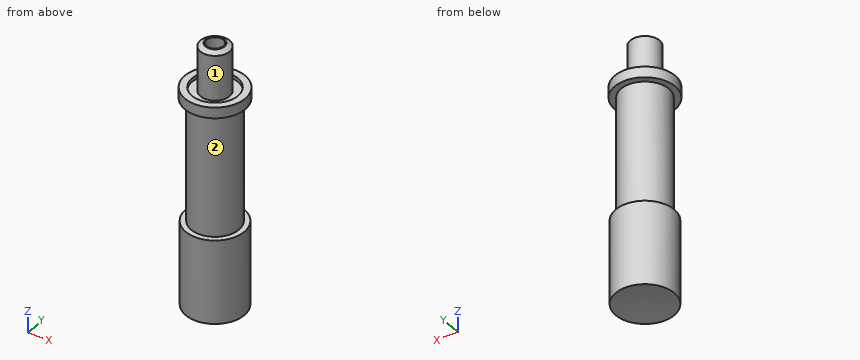
from build123d import *

# Parameters (mm, degrees)
CUT_EXTRUDE1_START = -10
SKETCH2_R          = 5
SKETCH2_R_2        = 2.45
CUT_EXTRUDE1_DEPTH = 10


with BuildPart() as part:
    # Sketch1 → Revolve1 (revolve)
    with BuildSketch(Plane(origin=(0, 0, 0), x_dir=(1, 0, 0), z_dir=(0, 1, 0))):
        with BuildLine():
            Line((0, 24.784048752), (0, 10.1))
            Line((0, 10.1), (0.6, 10.1))
            Line((0.6, 10.1), (0.7, 3.1))
            Line((0.7, 3.1), (0.79197487, 3.1))
            Line((0.79197487, 3.1), (1.225, 3.350011099))
            Line((1.225, 3.350011099), (1.225, 7.1))
            Line((1.225, 7.1), (1.925, 7.1))
            Line((1.925, 7.1), (1.925, 6.8))
            Line((1.925, 6.8), (2.525, 6.8))
            Line((2.525, 6.8), (2.525, 7.7))
            Line((2.525, 7.7), (2, 7.7))
            Line((2, 7.7), (2, 18))
            Line((2, 18), (2.45, 18))
            Line((2.45, 18), (2.45, 24))
            Line((2.45, 24), (4.2, 24))
            Line((4.2, 24), (4.2, 18))
            Line((4.2, 18), (5, 18))
            Line((5, 18), (5, 25))
            ThreePointArc((5, 25), (4.79361011, 25.404713607), (4.344827586, 25.475312026))
            ThreePointArc((4.344827586, 25.475312026), (2.199737011, 24.957944562), (0, 24.784048752))
        make_face()
    revolve(axis=Axis((0, 0, -25.5), (0, 0, 1)))

    # Sketch2 → Cut-Extrude1 (cut)
    with BuildSketch(Plane.XY.offset(-18).offset(CUT_EXTRUDE1_START)):
        Circle(SKETCH2_R)
        Circle(SKETCH2_R_2, mode=Mode.SUBTRACT)
    extrude(amount=CUT_EXTRUDE1_DEPTH, mode=Mode.SUBTRACT)


solid = part.part
Geometry: final body of the model. Coordinates: model frame, mm. Face numbers are marked on the shaded views. Give positions to 0.01 mm unless a question says otherwise; leave off trailing zeros. Order: outer loops, then holes, each group sorted by start corner. A loop starts at its lowest first (then second) coordinate and runs counter-clockwise, first axis right, second up. Notation, with made-up numbers: (84, -37) -> (132, -37) arc R19 ccw to (132, 0) -> close; hole circle Ø9 at (-35, -21.5). An arc over 180 degrees is marked (long way). Answer as a JSON object with one key per item and string values.
Q1. Material intervals for probe 1 along Y at (x, z) = (0, -7) (3 decimals); probe 2 along X at (y, z) = (-0.5, -8); probe 3 along Z at (x, y) = (0.2, 0.9), sorted ascending.
Entries:
{"probe 1": "y = -2.525 to -1.925, -1.225 to -0.644, 0.644 to 1.225, 1.925 to 2.525", "probe 2": "x = -1.94 to -0.38, 0.38 to 1.94", "probe 3": "z = -24.81 to -3.18"}
Q2. Section C-C (z = -19.25). Output: boundary loops of the cut face in (x, y), plus the area to 3 significant figures.
Entries:
{"outline": "circle Ø4.9 at (0, 0)", "area": "18.9 mm^2"}
Q3. First-contact query: pin 1 (3 mm diameter, centred on y = -2, z = -13, fed in from -X); pin 2 (3 mm diameter, centred on x = 0.5, z = -15.5, fed in from -Y); pin 3 (0.6 mm diameter, centred on x = -0.5, y = 0, fed in from +Z). Flat tips, straight axial feed; report the tip coordinate or a pass-through.
Entries:
{"pin 1": "stops at x = -1.94", "pin 2": "stops at y = -2", "pin 3": "stops at z = -3.1"}
Q4. Draft query along Z for the marked faces 1 and 2. Return one class per face: released by +Z, released by -Z, zero draft, split by the parting line, or undercut.
Entries:
{"face 1": "zero draft", "face 2": "undercut"}
Q5. Section A-A (z = -8). Output: boundary loops of the cut face in (x, y), plus the area to 3 significant figures.
Entries:
{"outline": "circle Ø4 at (0, 0); hole circle Ø1.26 at (0, 0)", "area": "11.3 mm^2"}
Q6. Section B-B (y = -1.45). Output: boundary loops of the cut face in (x, z).
Entries:
{"outline": "(-2.07, -7.7) -> (-1.38, -7.7) -> (-1.38, -18) -> (-1.97, -18) -> (-1.97, -25) arc R13.92 cw to (1.97, -25) -> (1.97, -18) -> (1.38, -18) -> (1.38, -7.7) -> (2.07, -7.7) -> (2.07, -6.8) -> (1.27, -6.8) -> (1.27, -7.1) -> (-1.27, -7.1) -> (-1.27, -6.8) -> (-2.07, -6.8) -> close"}
Q7. Section D-D (y = 1.65). Output: boundary loops of the cut face in (x, z).
Entries:
{"outline": "(-1.91, -7.7) -> (-1.13, -7.7) -> (-1.13, -18) -> (-1.81, -18) -> (-1.81, -25) arc R13.9 cw to (1.81, -25) -> (1.81, -18) -> (1.13, -18) -> (1.13, -7.7) -> (1.91, -7.7) -> (1.91, -6.8) -> (0.99, -6.8) -> (0.99, -7.1) -> (-0.99, -7.1) -> (-0.99, -6.8) -> (-1.91, -6.8) -> close"}
